```python
from build123d import *

# Parameters (mm, degrees)
F0_R     = 48.3453961675
F1_DEPTH = 50.8
F2_T     = -2.54


# Not quite as in the source:
# - a fillet or chamfer that OpenCascade refuses, or shapes differently, is made with other operations: its cross-section is extruded or revolved along the edge and cut away or added


with BuildPart() as f1:
    # F0 (on Front) → F1 (new body, symmetric)
    with BuildSketch(Plane.XZ):
        Circle(F0_R)
    extrude(amount=F1_DEPTH, both=True)

    # F2
    f2_openings = [f1.faces().sort_by_distance(p)[0] for p in [
        (0, 50.8, 0),
    ]]
    offset(amount=F2_T, openings=f2_openings)

    # F3: fillet of radius 5.08 on 3 edges, made by hand

    # F3_s1 → F3_t2 (revolve, cut)
    with BuildSketch(Plane.XY):
        with BuildLine():
            ThreePointArc((48.3453961675, 46.4005909488), (47.6648052188, 48.9405909488), (45.8053961675, 50.8))
            Line((45.8053961675, 50.8), (45.8561961675, 50.887988181))
            ThreePointArc((45.8561961675, 50.887988181), (47.0753961675, 50.9016), (48.3453961675, 50.9016))
            Line((48.3453961675, 50.9016), (48.4469961675, 50.8))
            Line((48.4469961675, 50.8), (48.4469961675, 46.4005909488))
            Line((48.4469961675, 46.4005909488), (48.3453961675, 46.4005909488))
        make_face()
    revolve(axis=Axis((0, 50.8, 0), (0, -1, 0)), mode=Mode.SUBTRACT)

    # F3_s3 → F3_t4 (revolve, cut)
    with BuildSketch(Plane.XY):
        with BuildLine():
            ThreePointArc((48.3453961675, -45.72), (46.857498616, -49.3121024484), (43.2653961675, -50.8))
            Line((43.2653961675, -50.8), (43.2653961675, -50.9016))
            Line((43.2653961675, -50.9016), (48.4469961675, -50.9016))
            Line((48.4469961675, -50.9016), (48.4469961675, -45.72))
            Line((48.4469961675, -45.72), (48.3453961675, -45.72))
        make_face()
    revolve(axis=Axis((0, -50.8, 0), (0, -1, 0)), mode=Mode.SUBTRACT)


solid = f1.part
```
Geometry: final body of the model. Coordinates: model frame, mm. Coordinates: 2 decimals unless noted, no trailing zeros. Order: outer loops, then holes, each group sorted by start corner. A loop starts at its lowest first (then second) coordinate and runs counter-clockwise, first axis right, second up.
Item 1: Contact query for flat-ended pins moving along their axis: P1, Ø5, axis at x = 34, y = -34.5, coming from the +Z side; P2, Ø6, axis at x = -2.5, z = 6, coming from the +Y side; P3, Ø2, axis at x = -35.5, y = -26.5, coming from the -Z side. Output: stop coordinate, or through.
Answer:
P1: stops at z = 36.67
P2: stops at y = -48.26
P3: stops at z = -33.87
Item 2: Section query B-B (z = 0). Output: boundary loops of the cut face in (x, y).
Answer:
outline: (-48.35, -45.72) arc R5.08 ccw to (-43.27, -50.8) - (43.27, -50.8) arc R5.08 ccw to (48.35, -45.72) - (48.35, 46.4) arc R5.08 ccw to (45.81, 50.8) - (45.81, -48.26) - (-45.81, -48.26) - (-45.81, 50.8) arc R5.08 ccw to (-48.35, 46.4) - close
Item 3: Material intervals for line 1 along Z through (x, y) = (0, 22); line 2 along Y through (x, z) = (-20.5, -18.5); line 3 along X through (y, z) = (21, -3.5), sorted ascending.
Answer:
line 1: z = -48.35 to -45.81, 45.81 to 48.35
line 2: y = -50.8 to -48.26
line 3: x = -48.22 to -45.67, 45.67 to 48.22
Item 4: Section query C-C (y = 7). Output: boundary loops of the cut face in (x, z).
Answer:
outline: circle Ø96.69 at (0, 0); hole circle Ø91.61 at (0, 0)
Item 5: Section query A-A (x = 0). Output: boundary loops of the cut face in (y, z).
Answer:
outline: (-50.8, -43.27) arc R5.08 ccw to (-45.72, -48.35) - (46.4, -48.35) arc R5.08 ccw to (50.8, -45.81) - (-48.26, -45.81) - (-48.26, 45.81) - (50.8, 45.81) arc R5.08 ccw to (46.4, 48.35) - (-45.72, 48.35) arc R5.08 ccw to (-50.8, 43.27) - close
Item 6: Draft query along Z for faces 1 (the face through (-1, -50.8, 1)), 2 (the face through (43.69, 0.58, 13.76)), 3 (the face through (-10.48, -0.305, -47.196)). Return one class per face: released by +Z, released by -Z, zero draft, split by the parting line, or undercut.
Answer:
face 1: zero draft
face 2: undercut
face 3: split by the parting line
